Geometry: final body of the model. Coordinates: model frame, mm. Face numbers are marked on the shaded views. Give positions to 0.01 mm unless a question says otherwise; leave off trailing zeros. Write each loop counter-clockwise with the first axis right and the second up, starting at its lowest first coordinate (ties: lowest second). Pieces come first, ordered by that corner, then holes.
Q1. Line query: line 1 (Z direction, x = -44.5, y = 5.5); line 2 (X direction, y = 6, z = -16); line 3 (Z direction, x = -29.5, y = 3.5). Output: solid intervals per line, ascending.
Q2. Section B-B (z = -16). Return the cut outline in (x, y).
Q3. Section D-D (y = 3). Return the cut outline in (x, z).
Q4. Mould query, pull axis Z, two halves, no side actions, for the marked faces 1, 2, 3 and 4. Classes: +Z half, -Z half, draft (parallel to the pull), parting line (faces both ways), or undercut.
Q5. Section A-A (x = -29). Return the cut outline in (y, z).
Q6. Pin query (flat end, axial travel): pin 1 Ø3.5 at (x, z) = (-13.5, 15) entering from -Y; pin 2 Ø2 at (y, z) = (2.5, 15) entering from +X. Return the tip coordinate at first contact, or that it passes through.
Q7. Section C-C (x = -44.5). Return the cut outline in (y, z), plus the area to 3 significant figures.
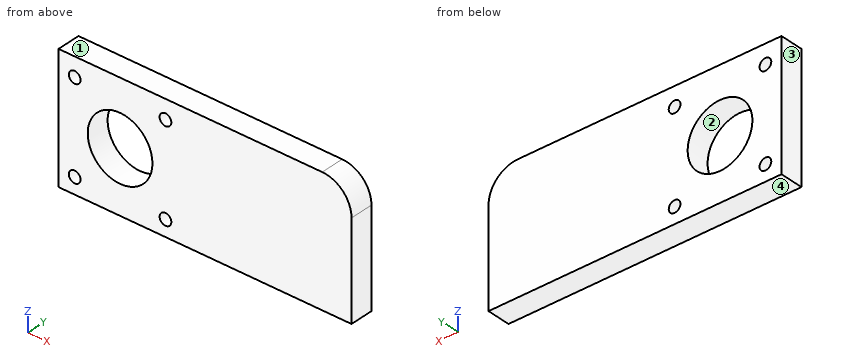
from build123d import *

# Parameters (mm, degrees)
SKETCH_1_R      = 11.05
SKETCH_1_R_2    = 2
EXTRUDE_1_DEPTH = 8


with BuildPart() as part:
    # Эскиз1 → Бобышка-Вытянуть1 (new body)
    with BuildSketch(Plane(origin=(0, 0, 0), x_dir=(1, 0, 0), z_dir=(0, 1, 0))):
        with BuildLine():
            Line((-50, -21.5), (40, -21.5))
            ThreePointArc((40, -21.5), (47.071067812, -18.571067812), (50, -11.5))
            Line((50, -11.5), (50, 21.5))
            Line((50, 21.5), (-50, 21.5))
            Line((-50, 21.5), (-50, -21.5))
        make_face()
        with Locations((-29, 0.5)):
            Circle(SKETCH_1_R, mode=Mode.SUBTRACT)
        with Locations((-13.5, -15)):
            Circle(SKETCH_1_R_2, mode=Mode.SUBTRACT)
        with Locations((-13.5, 16)):
            Circle(SKETCH_1_R_2, mode=Mode.SUBTRACT)
        with Locations((-44.5, -15)):
            Circle(SKETCH_1_R_2, mode=Mode.SUBTRACT)
        with Locations((-44.5, 16)):
            Circle(SKETCH_1_R_2, mode=Mode.SUBTRACT)
    extrude(amount=EXTRUDE_1_DEPTH)


solid = part.part
Computed:
1. line 1: z = -21.5 to -18, -14 to 13, 17 to 21.5
1. line 2: x = -50 to -46.5, -42.5 to -15.5, -11.5 to 50
1. line 3: z = -21.5 to -11.54, 10.54 to 21.5
2. outline: (-50, 0) - (-46.5, 0) - (-46.5, 8) - (-50, 8) - close; (-42.5, 0) - (-15.5, 0) - (-15.5, 8) - (-42.5, 8) - close; (-11.5, 0) - (50, 0) - (50, 8) - (-11.5, 8) - close
3. outline: (-50, -21.5) - (50, -21.5) - (50, 11.5) arc R10 ccw to (40, 21.5) - (-50, 21.5) - close; hole circle Ø4 at (-44.5, -16); hole circle Ø4 at (-44.5, 15); hole circle Ø22.1 at (-29, -0.5); hole circle Ø4 at (-13.5, -16); hole circle Ø4 at (-13.5, 15)
4. face 1: +Z half
4. face 2: undercut
4. face 3: draft
4. face 4: -Z half
5. outline: (0, -21.5) - (8, -21.5) - (8, -11.55) - (0, -11.55) - close; (0, 10.55) - (8, 10.55) - (8, 21.5) - (0, 21.5) - close
6. pin 1: passes through
6. pin 2: stops at x = 49.68
7. outline: (0, -21.5) - (8, -21.5) - (8, -18) - (0, -18) - close; (0, -14) - (8, -14) - (8, 13) - (0, 13) - close; (0, 17) - (8, 17) - (8, 21.5) - (0, 21.5) - close
7. area: 280 mm2
